Autodesk Inventor part; units mm, degrees
ref_plane "YZ Plane" through (0, 0, 0) normal (1, 0, 0) x (0, 1, 0)
ref_plane "XZ Plane" through (0, 0, 0) normal (0, 1, 0) x (-1, 0, 0)
ref_plane "XY Plane" through (0, 0, 0) normal (0, 0, 1) x (1, 0, 0)
sketch "Sketch1" plane through (0, 0, 0) normal (0, 0, 1) x (1, 0, 0)
  circle A0 centre (0, 0) radius 44
  dimension "d0" = 88
extrude "Extrusion1" add sketch "Sketch1" against normal blind 1
sketch "Sketch2" plane through (0, 0, 0) normal (0, 0, 1) x (1, 0, 0)
  circle A0 centre (0, 0) radius 44
  circle A1 centre (0, 38.1) radius 1.75
  circle A2 centre (0, -38.1) radius 1.75
  circle A3 centre (15.87, 0) radius 1.75
  circle A4 centre (-15.88, 0) radius 1.75
  circle A5 centre (-15.87, 25.4) radius 1.75
  circle A6 centre (-15.87, -25.4) radius 1.75
  circle A7 centre (15.87, 25.4) radius 1.75
  circle A8 centre (15.87, -25.4) radius 1.75
  dimension "d4" = 3.5
  dimension "d6" = 3.5
  dimension "d7" = 76.2
  dimension "d8" = 38.1
  dimension "d9" = 3.5
  dimension "d10" = 3.5
  dimension "d11" = 31.75
  dimension "d12" = 15.87
  dimension "d13" = 3.5
  dimension "d14" = 3.5
  dimension "d15" = 3.5
  dimension "d16" = 3.5
  dimension "d17" = 25.4
  dimension "d18" = 25.4
  dimension "d19" = 25.4
  dimension "d20" = 25.4
  dimension "d21" = 15.87
  dimension "d22" = 15.87
  dimension "d23" = 15.87
  dimension "d24" = 15.87
hole "Hole2" at (-15.87, 25.4, 0) at (0, 38.1, 0) at (15.87, 25.4, 0) at (15.87, 0, 0) at (15.87, -25.4, 0) at (0, -38.1, 0) at (-15.87, -25.4, 0) at (-15.88, 0, 0) direction (0, 0, -1) diameter 3.5 end through all
sketch "Sketch4" plane through (0, 0, 0) normal (0, 0, 1) x (1, 0, 0)
  circle A0 centre (0, 0) radius 44
  line L0 (-4.7625, 15) -> (4.7625, 15)
  line L1 (4.7625, 15) -> (4.7625, 10.05)
  line L2 (4.7625, 10.05) -> (-4.7625, 10.05)
  line L3 (-4.7625, 10.05) -> (-4.7625, 15)
  line L4 (-4.7625, 9.95) -> (4.7625, 9.95)
  line L5 (4.7625, 9.95) -> (4.7625, 5.05)
  line L6 (4.7625, 5.05) -> (-4.7625, 5.05)
  line L7 (-4.7625, 5.05) -> (-4.7625, 9.95)
  line L8 (-4.7625, 4.95) -> (4.7625, 4.95)
  line L9 (4.7625, 4.95) -> (4.7625, 0.05)
  line L10 (4.7625, 0.05) -> (-4.7625, 0.05)
  line L11 (-4.7625, 0.05) -> (-4.7625, 4.95)
  line L12 (-4.7625, -0.05) -> (4.7625, -0.05)
  line L13 (4.7625, -0.05) -> (4.7625, -4.95)
  line L14 (4.7625, -4.95) -> (-4.7625, -4.95)
  line L15 (-4.7625, -4.95) -> (-4.7625, -0.05)
  line L16 (-4.7625, -5.05) -> (4.7625, -5.05)
  line L17 (4.7625, -5.05) -> (4.7625, -9.95)
  line L18 (4.7625, -9.95) -> (-4.7625, -9.95)
  line L19 (-4.7625, -9.95) -> (-4.7625, -5.05)
  line L20 (-4.7625, -10.05) -> (4.7625, -10.05)
  line L21 (4.7625, -10.05) -> (4.7625, -15)
  line L22 (4.7625, -15) -> (-4.7625, -15)
  line L23 (-4.7625, -15) -> (-4.7625, -10.05)
  dimension "d53" = 9.525
  dimension "d55" = 4.95
  dimension "d56" = 15
  dimension "d57" = 4.7625
  dimension "d58" = 4.9
  dimension "d59" = 9.525
  dimension "d60" = 4.7625
  dimension "d61" = 9.95
  dimension "d62" = 4.9
  dimension "d63" = 0.05
  dimension "d64" = 9.525
  dimension "d65" = 4.7625
  dimension "d66" = 9.525
  dimension "d67" = 4.7625
  dimension "d68" = 4.9
  dimension "d69" = 0.05
  dimension "d70" = 4.9
  dimension "d71" = 9.525
  dimension "d72" = 4.7625
  dimension "d73" = 5.05
  dimension "d74" = 10.05
  dimension "d75" = 4.95
  dimension "d76" = 9.525
  dimension "d77" = 4.7625
extrude "Extrusion2" cut sketch "Sketch4" against normal up to next contours L0 L1 L2 L3 | L4 L5 L6 L7 | L8 L9 L10 L11 | L12 L13 L14 L15 | L16 L17 L18 L19 | L20 L21 L22 L23
equation "\"d6\" = d4"
equation "\"d9\" = d4"
equation "\"d10\" = d4"
equation "\"d13\" = d4"
equation "\"d14\" = d4"
equation "\"d15\" = d4"
equation "\"d16\" = d4"
equation "\"d21\" = d12"
equation "\"d22\" = d12"
equation "\"d23\" = d12"
equation "\"d24\" = d12"
equation "\"d37\" = Thickness"
equation "\"d57\" = 0.5 * d53"
equation "\"d59\" = d53"
equation "\"d60\" = 0.5 * d53"
equation "\"d64\" = d53"
equation "\"d65\" = 0.5 * d53"
equation "\"d66\" = d53"
equation "\"d67\" = 0.5 * d53"
equation "\"d71\" = d53"
equation "\"d72\" = 0.5 * d53"
equation "\"d76\" = d53"
equation "\"d77\" = 0.5 * d53"
equation "\"BendRadius\" = Thickness"
equation "\"BendReliefWidth\" = Thickness"
equation "\"BendReliefDepth\" = 0.5 * Thickness"
equation "\"CornerReliefSize\" = 4 * Thickness"
equation "\"MinimumRemnant\" = 2 * Thickness"
equation "\"TransitionRadius\" = BendRadius"
equation "\"JacobiRadiusSize\" = BendRadius"
equation "\"GapSize\" = Thickness"
properties part number "Plate"
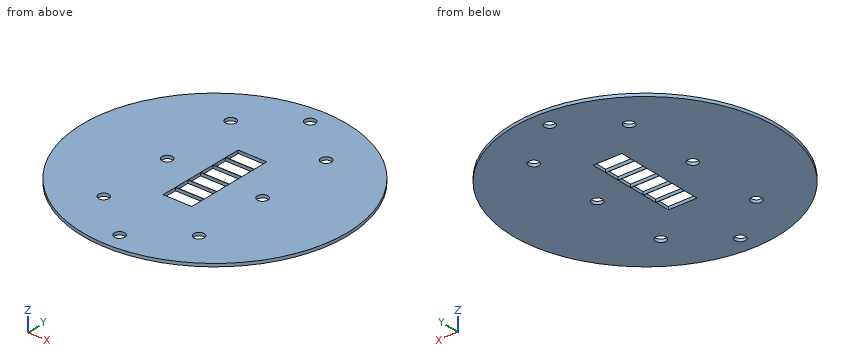
Input: part model. Units: mm. Frame: model coordinates. Coordinates: 2 decimals unless noted, no trailing zeros. Loops run counter-clockwise (first coordinate to the right, second up) from the corner with the lowest first, then second, coordinate; pieces in that order, holes last. Notation, with made-up numbers: M 43,26.25 L 63,26.25 A11 cw 63,40.25 Z; hole C 62.5,-13.5 d7. An arc over 180 degrees is marked long. Use a Markdown table: item, result. Add a question column.
1) Section C-C, the plane x = 15.87. Return the cut outline in (y, z).
2) Section D-D, the plane y = -25.4. Return the cut outline in (x, z).
3) Line query: L1, parallel to Y at x = 15.87, z = -0.6; L2, parallel to X at y = -25.4, z = -0.25; L3, parallel to X at y = 6, z = -0.65. Output: solid intervals per line, ascending. Write a range as from..to.
4) Section A-A, the plane z = -0.8. Give the number of separate pieces and of enclosed holes in the cut face, plus the area to 3 significant figures.
5) Section B-B, the plane y = 38.1. Return the cut outline in (x, z).
Answer below:
| question | item | result |
|---|---|---|
| 1 | outline | M -41.04,-1 L -27.15,-1 L -27.15,0 L -41.04,0 Z; M -23.65,-1 L -1.75,-1 L -1.75,0 L -23.65,0 Z; M 1.75,-1 L 23.65,-1 L 23.65,0 L 1.75,0 Z; M 27.15,-1 L 41.04,-1 L 41.04,0 L 27.15,0 Z |
| 2 | outline | M -35.93,-1 L -17.62,-1 L -17.62,0 L -35.93,0 Z; M -14.12,-1 L 14.12,-1 L 14.12,0 L -14.12,0 Z; M 17.62,-1 L 35.93,-1 L 35.93,0 L 17.62,0 Z |
| 3 | L1 | -41.04..-27.15, -23.65..-1.75, 1.75..23.65, 27.15..41.04 |
| 3 | L2 | -35.93..-17.62, -14.12..14.12, 17.62..35.93 |
| 3 | L3 | -43.59..-4.76, 4.76..43.59 |
| 4 | separate pieces | 1 |
| 4 | enclosed holes | 14 |
| 4 | area | 5,720 mm2 |
| 5 | outline | M -22.01,-1 L -1.75,-1 L -1.75,0 L -22.01,0 Z; M 1.75,-1 L 22.01,-1 L 22.01,0 L 1.75,0 Z |
